Verification items for this drawing (mm, ordinates from the low corner). Round coordinates to 2 decimals unless told otherwise and drop trailing zeros. Write each loop counter-clockwise with the first axis right and the second up, starting at its lowest first coordinate (ties: lowest second). Pieces come first, ordered by that corner, then holes. Notation, with made-up numbers: (-21.5, 87) -> (-4.5, 87) arc R23 cw to (-4.5, 97) -> close; hole circle Ø5 at (-32.5, 55.25). An arc over 180 degrees is marked (long way). One line per question, with ' | ' between items.
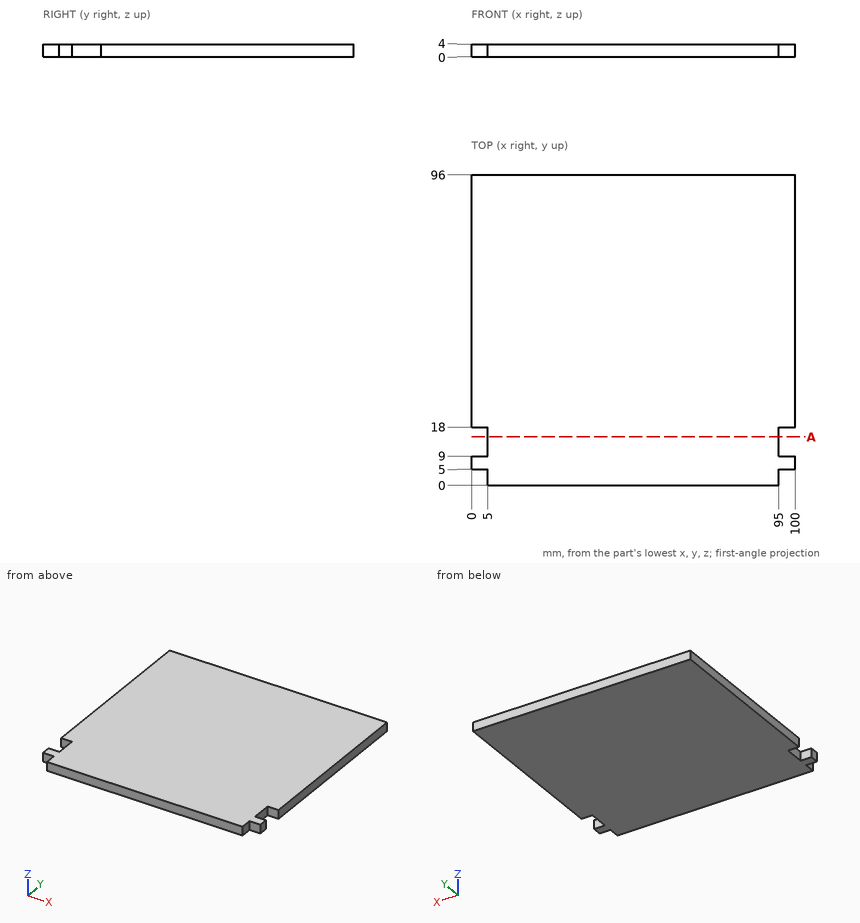
(1) Sectioned sample at A-A on y = 15. Record the cut outline in (x, z), then the cut area to 3 significant figures.
Resolved:
outline: (5, 0) -> (95, 0) -> (95, 4) -> (5, 4) -> close | area: 360 mm2
(2) Go/stop test with flat-tipped pins: pin 1 (2 mm diameter, centred on y = 1.5, z = 2, fed in from -X); pin 2 (2 mm diameter, centred on x = 96.5, z = 2, fed in from -Y); pin 3 (1.2 mm diameter, centred on y = 11.5, z = 2.5, fed in from +X). Record where each tip stops, or that it passes through.
Resolved:
pin 1: stops at x = 5 | pin 2: stops at y = 5 | pin 3: stops at x = 95
(3) Material ranges on line 1 (X direction, y = 12.5, z = 2.4), recorded low to high.
Resolved:
line 1: x = 5 to 95
